```python
from build123d import *

# Parameters (mm, degrees)
SKETCH1_R           = 16
SKETCH1_R_2         = 15
BOSS_EXTRUDE1_DEPTH = 64
CUT_EXTRUDE1_DEPTH  = 4
CUT_EXTRUDE2_DEPTH  = 4


with BuildPart() as part:
    # Sketch1 → Boss-Extrude1 (new body)
    with BuildSketch(Plane(origin=(0, 0, 0), x_dir=(1, 0, 0), z_dir=(0, 1, 0))):
        Circle(SKETCH1_R)
        Circle(SKETCH1_R_2, mode=Mode.SUBTRACT)
    extrude(amount=BOSS_EXTRUDE1_DEPTH)

    # Sketch2 → Cut-Extrude1 (cut)
    with BuildSketch(Plane(origin=(0, 64, 0), x_dir=(1, 0, 0), z_dir=(0, 1, 0))):
        Polygon((0, 0), (0, 5.5), (-16.81016258, 5.5), (-16.81016258, -5.5), (0, -5.5), align=None)
    extrude(amount=-CUT_EXTRUDE1_DEPTH, mode=Mode.SUBTRACT)

    # Sketch3 → Cut-Extrude2 (cut)
    with BuildSketch(Plane.XZ):
        Polygon((0, 0), (0, 5.5), (-17.011405804, 5.5), (-17.011405804, -5.5), (0, -5.5), align=None)
    extrude(amount=-CUT_EXTRUDE2_DEPTH, mode=Mode.SUBTRACT)


solid = part.part
```
The model under review builds one solid part; all positions refer to its coordinate system, in mm. A direction names the side the tool comes from. Give positions to 0.01 mm unless a question says otherwise; leave off trailing zeros. Write each loop counter-clockwise with the first axis right and the second up, starting at its lowest first coordinate (ties: lowest second). Pieces come first, ordered by that corner, then holes.
(1) Tool access review of faces 1 (the cylindrical face through (13.856, 31.552, 5.745)), 2 (the flat face through (-15.2, 4, 0.1)): name each direction out of +Z, -Z, +X, -X, +Y, -Y from which nothing blocks a thin tool from reaching the whole face with its end or side.
(2) Consider section B-B, the plane z = 0. Give the boundary of the cut face in (x, y), and give its area (3 significant figures).
(3) Consider section A-A, the plane x = 0. Give the boundary of the cut face in (y, z), and give its area (3 significant figures).
(4) Consider section C-C, the plane y = 53. Give the boundary of the cut face in (x, z), and give its area (3 significant figures).
(5) For P1, Ø0.9, axis at x = -14, y = 1, coming from the -Z side; P2, Ø0.5, axis at x = -14.5, y = 61.5, coming from the -Z side; P3, Ø1.2, axis at x = -14.5, y = 61.5, coming from the +Z side, all flat-tipped, find the tip position at first contact; note any pin that passes through.
(6) The part is to be moulded in two halves that separate along Z. For faces 3 (the flat face through (11.9, 64, 9.4)), 4 (the cylindrical face through (14.78, 31.55, 6.13)), 5 (the flat face through (-15.2, 60, -0.1)), say which applies: released by +Z, released by -Z, zero draft, split by the parting line, or undercut.
(7) To check wall thickness, follow L1, parallel to Z at x = 0, y = 35; L2, parallel to Z at x = -13, y = 58.5; L3, parallel to X at y = 4, z = -7. State the ranges of each line that lie inside material, in increasing order.
Returned:
1. face 1: +Y, -Y
1. face 2: -X, -Y
2. outline: (-16, 4) - (-15, 4) - (-15, 60) - (-16, 60) - close; (15, 0) - (16, 0) - (16, 64) - (15, 64) - close
2. area: 120 mm2
3. outline: (0, -16) - (64, -16) - (64, -15) - (0, -15) - close; (0, 15) - (64, 15) - (64, 16) - (0, 16) - close
3. area: 128 mm2
4. outline: circle Ø32 at (0, 0); hole circle Ø30 at (0, 0)
4. area: 97.4 mm2
5. P1: stops at z = -8.51
5. P2: stops at z = -7.28
5. P3: stops at z = 7.92
6. face 3: zero draft
6. face 4: split by the parting line
6. face 5: undercut
7. L1: z = -16 to -15, 15 to 16
7. L2: z = -9.33 to -7.48, 7.48 to 9.33
7. L3: x = -14.39 to -13.27, 13.27 to 14.39
